Read the model definition and answer for the solid it produces. Units are mm, in the model's axes. Face numbers are marked on the shaded views. A direction names the side the tool comes from. Round coordinates to 2 decimals unless told otherwise and drop trailing zeros. Order: outer loops, then holes, each group sorted by start corner. A loop starts at its lowest first (then second) coordinate and runs counter-clockwise, first axis right, second up. Notation, with made-up numbers: (50, -38.5) -> (69, -38.5) arc R36 ccw to (69, -4.5) -> close; hole circle Ø3 at (47.5, 49). An arc over 180 degrees is marked (long way). Answer as a JSON object with one key per item and string values. Group by question number.
Item 1: Section A-A, the plane y = 15 is taken. Write down the section's boundary in (x, z), plus the area to 3 significant figures.
Item 2: For the marked faces 1, 2 and 3, determine the directions among +Z, -Z, +X, -X, +Y, -Y from which every point of the face is accessible in a straight line to the end or side of a thin tool.
Item 3: Section B-B, the plane x = 12 is taken. Write down the section's boundary in (y, z), plus the area to 3 significant figures.
Item 4: Section C-C, the plane z = 24 is taken. Write down the section's boundary in (x, y), plus the area to 3 significant figures.
Item 5: The mould has two halves that part along X. Classify the marked faces 4, 5 and 6: pulls with the +X half, pulls with the -X half, needs draft (parallel to the pull), parting line crosses it, or undercut.
Item 6: Consider probe 1 along X at (y, z) = (22, 20.75); probe 2 along Z at (x, y) = (-16, 22); probe 3 along Z at (x, y) = (-16, 20.75). Determine where each line is inside the solid, lowest interval first. Write a range as from..to.
Item 7: Section D-D, the plane x = -19 is taken. Write down the section's boundary in (y, z), plus the area to 3 significant figures.
Item 8: Given P1, Ø3, axis at x = 16, z = 20.5, coming from the +Y side; P2, Ø3.5, axis at x = -16, z = 20.75, coming from the -Y side; P3, Ø10, axis at x = -1, y = 6.5, coming from the +Z side; P4, Ø4.5, axis at x = -0.5, y = 24, coming from the -Z side, each flat-ended and moving along its own axis, determine where each tip first touches the part or whether it passes through.
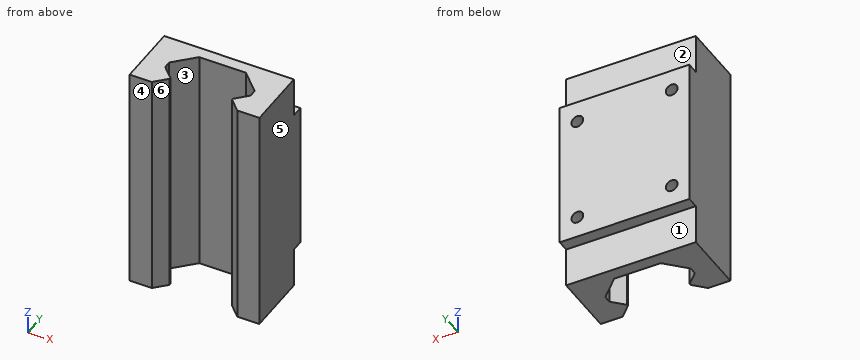
Autodesk Inventor part; units mm, degrees
ref_plane "YZ Plane" through (0, 0, 0) normal (1, 0, 0) x (0, 1, 0)
ref_plane "XZ Plane" through (0, 0, 0) normal (0, 1, 0) x (-1, 0, 0)
ref_plane "XY Plane" through (0, 0, 0) normal (0, 0, 1) x (1, 0, 0)
sketch "Sketch1" plane through (0, 0, 0) normal (0, 0, 1) x (1, 0, 0)
  line L0 (0, 0) -> (-22, 0)
  line L1 (-22, 0) -> (-22, 0)
  line L2 (-22, 0) -> (-14.5, 0)
  line L3 (-22, 0) -> (-22, 25.4)
  line L4 (-22, 25.4) -> (0, 25.4)
  line L5 (-29.0722, -4.6) -> (-18.7593, -4.6) construction
  line L6 (-22, 0) -> (0, 0) construction
  line L7 (0, 0) -> (22, 0) construction
  line L8 (0, -10.6) -> (0, 31.4) construction
  line L9 (0, -4.6) -> (0, 12.9) construction
  line L10 (0, -4.6) -> (-10, -4.6) construction
  line L11 (0, -4.6) -> (10, -4.6) construction
  line L12 (-10, -4.6) -> (-10, 0) construction
  line L13 (-10, 0) -> (-6.1, 3.9) construction
  line L14 (-6.1, 3.9) -> (-6.1, 4.4) construction
  line L15 (-6.1, 4.4) -> (-10, 8.3) construction
  line L16 (-10, 8.3) -> (-10, 10.8) construction
  line L17 (-10, 10.8) -> (-7.9, 12.9) construction
  line L18 (-7.9, 12.9) -> (0, 12.9) construction
  line L19 (10, 0) -> (6.1, 3.9) construction
  line L20 (6.1, 3.9) -> (6.1, 4.4) construction
  line L21 (6.1, 4.4) -> (10, 8.3) construction
  line L22 (10, 8.3) -> (10, 10.8) construction
  line L23 (10, 10.8) -> (7.9, 12.9) construction
  line L24 (10, -4.6) -> (10, 0) construction
  line L25 (7.9, 12.9) -> (0, 12.9) construction
  line L26 (-14.5, 8.3) -> (-14.5, 10.8)
  line L27 (-14.5, 10.8) -> (-7.9, 17.4)
  line L28 (-7.9, 17.4) -> (0, 17.4)
  line L29 (-14.5, 0) -> (-10.6, 3.9)
  line L30 (-10.6, 3.9) -> (-10.6, 4.4)
  line L31 (-10.6, 4.4) -> (-14.5, 8.3)
  line L32 (-10.6, 3.9) -> (-6.1, 3.9) construction
  line L33 (-10, 8.3) -> (-14.5, 8.3) construction
  line L34 (22, 0) -> (14.5, 0)
  line L35 (22, 0) -> (22, 25.4)
  line L36 (22, 25.4) -> (0, 25.4)
  line L37 (14.5, 8.3) -> (14.5, 10.8)
  line L38 (14.5, 10.8) -> (7.9, 17.4)
  line L39 (7.9, 17.4) -> (0, 17.4)
  line L40 (14.5, 0) -> (10.6, 3.9)
  line L41 (10.6, 3.9) -> (10.6, 4.4)
  line L42 (10.6, 4.4) -> (14.5, 8.3)
  point P0 (-3.95, 17.4)
  dimension "d0" = 4.6
  dimension "d1" = 44
  dimension "d3" = 17.5
  dimension "d4" = 20
  dimension "d5" = 4.6
  dimension "d6" = 8.5
  dimension "d7" = 135
  dimension "d8" = 0.5
  dimension "d9" = 135
  dimension "d10" = 2.5
  dimension "d11" = 7.5
  dimension "d12" = 25.4
  dimension "d13" = 45
  dimension "d14" = 135
  dimension "d15" = 2.5
  dimension "d16" = 0.5
  dimension "d17" = 135
  dimension "d19" = 4.5
extrude "Extrusion1" add sketch "Sketch1" along normal blind 77.5
sketch "Sketch2" plane through (-22, 25.4, 0) normal (0, 1, 0) x (1, 0, 0)
  circle A0 centre (6, -20.75) radius 2
  circle A1 centre (6, -56.75) radius 2
  line L0 (6, -20.75) -> (6, -56.75)
  circle A2 centre (38, -20.75) radius 2
  circle A3 centre (38, -56.75) radius 2
  line L1 (38, -20.75) -> (38, -56.75) construction
  line L2 (22, 0) -> (22, -77.5) construction
  line L3 (44, -77.5) -> (0, -77.5) construction
  line L4 (38, -38.75) -> (22, -38.75) construction
  line L5 (6, -38.75) -> (22, -38.75) construction
  line L6 (0, 0) -> (0, -77.5) construction
  line L7 (44, -64) -> (0, -64) construction
  line L8 (0, -64) -> (0, -13.5) construction
  line L9 (0, -13.5) -> (44, -13.5) construction
  line L10 (44, -13.5) -> (44, -64) construction
  line L11 (44, -64) -> (0, -13.5) construction
  line L12 (0, -64) -> (44, -13.5) construction
  line L13 (44, 0) -> (44, -77.5)
  line L14 (0, -13.5) -> (44, -13.5)
  line L15 (44, -13.5) -> (44, 0)
  line L16 (44, 0) -> (0, 0)
  line L17 (0, 0) -> (0, -13.5)
  line L18 (0, -64) -> (44, -64)
  line L19 (44, -64) -> (44, -77.5)
  line L20 (44, -77.5) -> (0, -77.5)
  line L21 (0, -77.5) -> (0, -64)
  point P0 (7.5, -77.5)
  dimension "d22" = 36
  dimension "d23" = 4
  dimension "d24" = 4
  dimension "d25" = 36
  dimension "d26" = 4
  dimension "d27" = 4
  dimension "d29" = 32
  dimension "d30" = 50.5
extrude "Extrusion2" cut sketch "Sketch2" against normal blind 8 contours A0 | A1 | A2 | A3
extrude "Extrusion3" cut sketch "Sketch2" against normal blind 4 contours L13 L20 L21 L18 | L13 L14 L17 L16
equation "\"d15\" = d10"
equation "\"d16\" = d8"
properties part number "HGH20CA Slider Block"
Values found:
{
 "1": {"outline": "(-22, 0) -> (-10.3, 0) -> (-10.3, 77.5) -> (-22, 77.5) -> close; (10.3, 0) -> (22, 0) -> (22, 77.5) -> (10.3, 77.5) -> close", "area": "1,810 mm2"},
 "2": {"face 1": "-Z, +X, -X, +Y", "face 2": "+Z, +X, -X, +Y", "face 3": "+Z, -Z"},
 "3": {"outline": "(2.5, 0) -> (5.8, 0) -> (5.8, 77.5) -> (2.5, 77.5) -> close; (13.3, 0) -> (21.4, 0) -> (21.4, 13.5) -> (25.4, 13.5) -> (25.4, 64) -> (21.4, 64) -> (21.4, 77.5) -> (13.3, 77.5) -> close", "area": "1,090 mm2"},
 "4": {"outline": "(-22, 0) -> (-14.5, 0) -> (-10.6, 3.9) -> (-10.6, 4.4) -> (-14.5, 8.3) -> (-14.5, 10.8) -> (-7.9, 17.4) -> (7.9, 17.4) -> (14.5, 10.8) -> (14.5, 8.3) -> (10.6, 4.4) -> (10.6, 3.9) -> (14.5, 0) -> (22, 0) -> (22, 25.4) -> (-22, 25.4) -> close", "area": "691 mm2"},
 "5": {"face 4": "needs draft", "face 5": "pulls with the +X half", "face 6": "undercut"},
 "6": {"probe 1": "-22..-18, -14..14, 18..22", "probe 2": "13.5..18.75, 22.75..54.75, 58.75..64", "probe 3": "0..18.75, 22.75..54.75, 58.75..77.5"},
 "7": {"outline": "(0, 0) -> (21.4, 0) -> (21.4, 13.5) -> (25.4, 13.5) -> (25.4, 64) -> (21.4, 64) -> (21.4, 77.5) -> (0, 77.5) -> close", "area": "1,860 mm2"},
 "8": {"P1": "y = 17.4", "P2": "y = 0", "P3": "through", "P4": "z = 13.5"}
}
